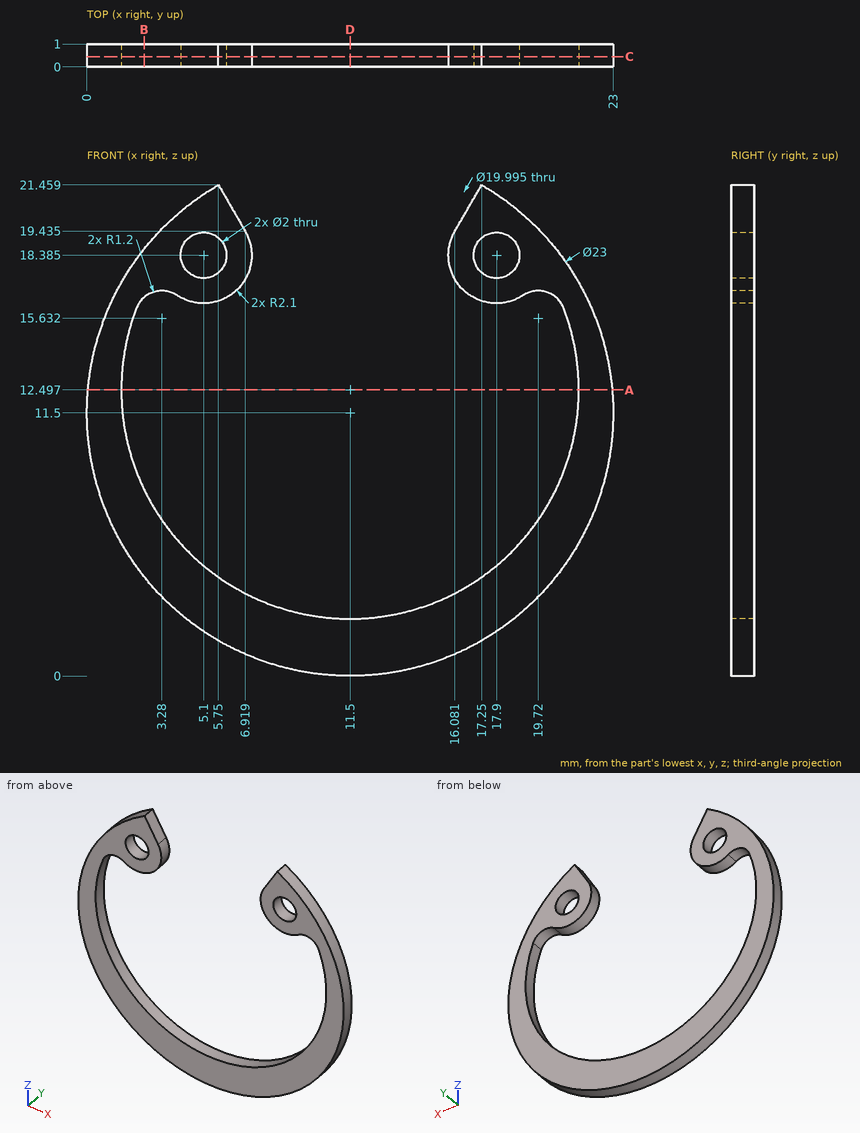
Verification items for this drawing (mm, ordinates from the low corner). Coordinates: 2 decimals unless noted, no trailing zeros. Order: outer loops, then holes, each group sorted by start corner. A loop starts at its lowest first (then second) coordinate and runs counter-clockwise, first axis right, second up. Notation, with made-up numbers: (36.25, -18.75) -> (76.25, -18.75) arc R21 ccw to (76.25, 8.25) -> close; hole circle Ø10 at (86, -31.5). An arc over 180 degrees is marked (long way). Put each result on its own line as item: value. Start each with the question number.
1. Material ranges on L1, parallel to X at y = 0.35, z = 18.5 (1 decimal); L2, parallel to Z at x = 16.25, y = 0.75 (1 decimal); L3, parallel to X at y = 0.7, z = 4 (1 decimal), recorded low to high. Write a range as [from, to].
2. Cross-section at C-C, the plane y = 0.45. Count the separate pieces of the cut face and the enclosed holes in it.
3. Cross-section at A-A, the plane z = 12.5. Record the boundary of the cut face in (x, y).
4. Go/stop test with a flat-tipped pin: pin 1 Ø1.8 at (x, z) = (5.1, 18.38) entering from -Y. Record where the tip stops, or that it passes through.
5. Cross-section at D-D, the plane x = 11.5. Record the boundary of the cut face in (y, z).
6. Cross-section at B-B, the plane x = 2.5. Record the boundary of the cut face in (y, z) (1 decimal).
Computed:
1. L1: [2.4, 4.1], [6.1, 7.2], [15.8, 16.9], [18.9, 20.6]
1. L2: [1, 3.7], [17.1, 19.7]
1. L3: [2.8, 6.2], [16.8, 20.2]
2. separate pieces: 1
2. enclosed holes: 2
3. outline: (0.04, 0) -> (1.5, 0) -> (1.5, 1) -> (0.04, 1) -> close; (21.5, 0) -> (22.96, 0) -> (22.96, 1) -> (21.5, 1) -> close
4. pin 1: through
5. outline: (0, 0) -> (1, 0) -> (1, 2.5) -> (0, 2.5) -> close
6. outline: (0, 4.3) -> (1, 4.3) -> (1, 8.1) -> (0, 8.1) -> close; (0, 16.5) -> (1, 16.5) -> (1, 18.7) -> (0, 18.7) -> close
